Autodesk Inventor part; units mm, degrees
ref_plane "YZ Plane" through (0, 0, 0) normal (1, 0, 0) x (0, 1, 0)
ref_plane "XZ Plane" through (0, 0, 0) normal (0, 1, 0) x (-1, 0, 0)
ref_plane "XY Plane" through (0, 0, 0) normal (0, 0, 1) x (1, 0, 0)
sketch "Sketch1" plane through (0, 0, 0) normal (1, 0, 0) x (0, 1, 0)
  line L0 (45.2604, 28.0988) -> (45.2604, -22.7012)
  line L1 (45.2604, -22.7012) -> (19.8604, -22.7012)
  line L2 (19.8604, -22.7012) -> (-56.3396, 2.6988)
  line L3 (-56.3396, 2.6988) -> (-56.3396, 28.0988)
  line L4 (45.2604, 28.0988) -> (-56.3396, 28.0988)
  point P0 (0, 0)
  dimension "d0" = 50.8
  dimension "d1" = 25.4
  dimension "d2" = 76.2
  dimension "d3" = 25.4
extrude "Extrusion1" add sketch "Sketch1" along normal blind 19.05
sketch "Sketch2" plane through (0, 45.2604, 28.0988) normal (0, 1, 0) x (1, 0, 0)
  line L0 (19.05, 50.8) -> (19.05, 0)
  line L1 (19.05, 0) -> (12.7, 0)
  line L2 (12.7, 0) -> (12.7, 12.7)
  line L3 (12.7, 12.7) -> (19.05, 12.7)
  line L4 (19.05, 12.7) -> (19.05, 0)
  line L5 (0, 0) -> (19.05, 0)
  line L6 (0, 0) -> (6.35, 0)
  line L7 (6.35, 0) -> (6.35, 12.7)
  line L8 (6.35, 12.7) -> (0, 12.7)
  line L9 (0, 12.7) -> (0, 0)
  point P0 (0, 28.0988)
  dimension "d6" = 6.35
  dimension "d7" = 12.7
  dimension "d8" = 6.35
extrude "Extrusion2" cut sketch "Sketch2" against normal blind 101.6
fillet "Fillet1" radius 3.175 2 edges at (19.05, -18.2396, -10.0012) (19.05, 32.5604, -22.7012)
equation "\"d9\" = d3 + d2"
properties part number "Right Leg, Side Partt"
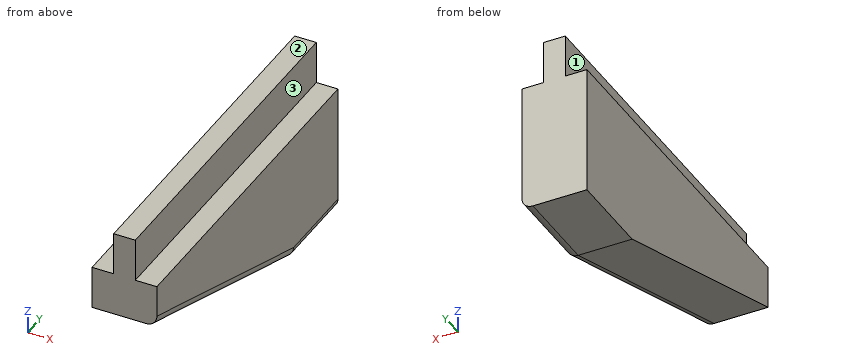
For this review, take the finished solid that the model builds, in its own axes (mm). Face numbers are marked on the shaded views. A direction names the side the tool comes from. Coordinates: 2 decimals unless noted, no trailing zeros. Order: outer loops, then holes, each group sorted by start corner. A loop starts at its lowest first (then second) coordinate and runs counter-clockwise, first axis right, second up. Notation, with made-up numbers: (-10.75, 76) -> (47.25, 76) arc R8 ccw to (47.25, 84) -> close; hole circle Ø2 at (-22, 9.5). An arc over 180 degrees is marked (long way). Return JSON: item names as keys, results as strings.
1. We need section B-B on x = 5.25. Write out the cut boundary in (y, z), and give its area (3 significant figures).
Answer block:
{"outline": "(-56.34, 2.7) -> (19.86, -22.7) -> (45.26, -22.7) -> (45.26, 15.4) -> (-56.34, 15.4) -> close", "area": "2,900 mm²"}
2. We need section D-D on x = 11.5. Write out the cut boundary in (y, z).
Answer block:
{"outline": "(-56.34, 2.7) -> (19.86, -22.7) -> (45.26, -22.7) -> (45.26, 28.1) -> (-56.34, 28.1) -> close"}
3. We need section A-A on y = 34. Write out the cut boundary in (x, z) (3 decimals), and give its area (3 significant figures).
Answer block:
{"outline": "(0, -22.701) -> (15.875, -22.701) arc R3.175 ccw to (19.05, -19.526) -> (19.05, 15.399) -> (12.7, 15.399) -> (12.7, 28.099) -> (6.35, 28.099) -> (6.35, 15.399) -> (0, 15.399) -> close", "area": "804 mm²"}
4. For line 1 (Z direction, x = 13.25, y = 24.5); line 2 (X direction, y = -11.5, z = 24); line 3 (Z direction, x = 11.25, y = 3.5), list the stretches that pass through material, from the lowest coordinate up. Write a range as from..to.
Answer block:
{"line 1": "-22.7..15.4", "line 2": "6.35..12.7", "line 3": "-17.25..28.1"}
5. For pin 1 Ø10 at (y, z) = (3.5, -8.5) entering from -X; pin 2 Ø3 at (x, y) = (15, -30) entering from +Z; pin 3 Ø10 at (y, z) = (-25.5, 21.5) entering from -X; pin 4 Ø1 at (x, y) = (6.5, -34.5) entering from -Z, all flat-tipped, find the tip position at first contact; note any pin that passes through.
Answer block:
{"pin 1": "x = 0", "pin 2": "z = 15.4", "pin 3": "x = 6.35", "pin 4": "z = -4.75"}
6. Machinability: for the marked faces 1, 2 and 3, which of the approach directions +Z, -Z, +X, -X, +Y, -Y give a long, thin tool a straight path to every point of the face, cutting with its end or side? Answer none if there is none.
Answer block:
{"face 1": "+Z, -X, +Y, -Y", "face 2": "+Z, +X, -X, +Y, -Y", "face 3": "+Z, +X, +Y, -Y"}
7. We need section C-C on z = 18. Write out the cut boundary in (x, y).
Answer block:
{"outline": "(6.35, -56.34) -> (12.7, -56.34) -> (12.7, 45.26) -> (6.35, 45.26) -> close"}
